Source: CAD feature listing. Evaluate the final solid. Frame: model axes, mm. A direction names the side the tool comes from. Coordinates: 2 decimals unless noted, no trailing zeros. Write each loop counter-clockwise with the first axis right and the second up, starting at its lowest first coordinate (ties: lowest second). Pieces come first, ordered by that corner, then holes. Notation, with made-up numbers: M 85.25,-15 L 117.25,-15 A19 cw 117.25,-7 Z; hole C 1,41 d4. An arc over 180 degrees is marked long. Write item = value, one per line. Start each with the question number.
1. Access query for faces 1 (the face through (-43.714, 6.409, -23.412)), 2 (the face through (-38, 6, -17.55)), 3 (the face through (-47.6, 7, -6)). Directions: +Z, -Z, +X, -X, +Y, -Y. A direction counts if a zero-diameter tool reaches every point of the face in a straight line with its end or side. Return the directions, or none.
2. Section query A-A (z = 23.75). Output: boundary loops of the cut face in (x, y).
3. Pull-direction query (X, two-part tool) for faces 4 (the face through (-43.714, 6.409, 24.088)), 5 (the face through (-44, 12, 0)), 6 (the face through (-47.6, 7, 5)); classes: pulls with the +X half, pulls with the -X half, needs draft (parallel to the pull), parting line crosses it, or undercut.
4. Pin query (flat end, axial travel): pin 1 Ø6.5 at (y, z) = (5, -6) entering from +X; pin 2 Ø4.5 at (x, z) = (-41.14, -23.75) entering from +Y; pin 3 Ø1 at (x, y) = (-43, 2.5) entering from +Z; pin 4 Ø3 at (y, z) = (10, 5.5) entering from -X. Return the tip coordinate at first contact, or that it passes through.
5. Section query D-D (x = -46.5). Output: boundary loops of the cut face in (y, z), then the cut area to 3 significant figures.
6. Line query: line 1 along Z through (x, y) = (-41, 9); line 2 along Z through (x, y) = (-42.75, 7.75); line 3 along Y through (x, z) = (-42.75, 3). Output: solid intervals per line, ascending.
7. Section query C-C (y = 4). Output: boundary loops of the cut face in (x, z), then the cut area to 3 significant figures.
8. Section query B-B (x = -39.25). Output: boundary loops of the cut face in (y, z), then the cut area to 3 significant figures.
```python
from build123d import *

# Parameters (mm, degrees)
SKETCH_1_R          = 2.6
EXTRUDE_1_DEPTH     = 13
SKETCH_2_W          = 0.6
SKETCH_2_H          = 35.1
CUT_EXTRUDE_1_DEPTH = 23
CUT_EXTRUDE_2_DEPTH = 6


with BuildPart() as part:
    # 草图1 → 凸台-拉伸1 (new body)
    with BuildSketch(Plane(origin=(0, 0, 0), x_dir=(1, 0, 0), z_dir=(0, 1, 0))):
        with BuildLine():
            Line((-33.760275315, -17.55), (-41, -17.55))
            Line((-41, -17.55), (-41, 17.55))
            Line((-41, 17.55), (-33.760275315, 17.55))
            ThreePointArc((-33.760275315, 17.55), (-36.796000438, 25.438985546), (-40.910253672, 32.823065739))
            ThreePointArc((-40.910253672, 32.823065739), (-52.45, 0), (-40.910253672, -32.823065739))
            ThreePointArc((-40.910253672, -32.823065739), (-36.796000438, -25.438985546), (-33.760275315, -17.55))
        make_face()
        with Locations(Location((-41.13620668, -23.75, 0), (0, 0, 90))):
            Circle(SKETCH_1_R, mode=Mode.SUBTRACT)
        with Locations(Location((-41.13620668, 23.75, 0), (0, 0, 90))):
            Circle(SKETCH_1_R, mode=Mode.SUBTRACT)
        with Locations(Location((-47.5, 0, 0), (0, 0, 90))):
            Circle(SKETCH_1_R, mode=Mode.SUBTRACT)
    extrude(amount=EXTRUDE_1_DEPTH)

    # 草图2 → 切除-拉伸1 (cut)
    with BuildSketch(Plane(origin=(0, 13, 0), x_dir=(1, 0, 0), z_dir=(0, 1, 0))):
        with Locations((-41.3, 0)):
            Rectangle(SKETCH_2_W, SKETCH_2_H)
    extrude(amount=-CUT_EXTRUDE_1_DEPTH, mode=Mode.SUBTRACT)

    # 草图3 → 切除-拉伸2 (cut)
    with BuildSketch(Plane(origin=(-41.6, 0, 0), x_dir=(0, 0, -1), z_dir=(1, 0, 0))):
        with BuildLine():
            Line((-5, 12), (5, 12))
            ThreePointArc((5, 12), (10, 7), (5, 2))
            Line((5, 2), (-5, 2))
            ThreePointArc((-5, 2), (-10, 7), (-5, 12))
        make_face()
    extrude(amount=-CUT_EXTRUDE_2_DEPTH, mode=Mode.SUBTRACT)


solid = part.part
```
Results are:
q1.face_1 = +Y, -Y
q1.face_2 = +X, +Y, -Y
q1.face_3 = +X
q2.outline = M -46.76,0 L -43.74,0 L -43.74,13 L -46.76,13 Z; M -38.54,0 L -36.04,0 L -36.04,13 L -38.54,13 Z
q3.face_4 = undercut
q3.face_5 = needs draft
q3.face_6 = pulls with the +X half
q4.pin_1 = -41.6
q4.pin_2 = through
q4.pin_3 = 30.74
q4.pin_4 = -52.3
q5.outline = M 0,-24.26 L 13,-24.26 L 13,-2.4 L 12,-2.4 L 12,-5 A5 cw 2,-5 L 2,-2.4 L 0,-2.4 Z; M 0,2.4 L 2,2.4 L 2,5 A5 cw 12,5 L 12,2.4 L 13,2.4 L 13,24.26 L 0,24.26 Z
q5.area = 438 mm^2
q6.line_1 = -32.71 to -26.35, -21.15 to -17.55, 17.55 to 21.15, 26.35 to 32.71
q6.line_2 = -30.39 to -25.79, -21.71 to -9.94, 9.94 to 21.71, 25.79 to 30.39
q6.line_3 = 0 to 2, 12 to 13
q7.outline = M -47.6,-9 L -47.6,-2.6 A2.6 cw -47.6,2.6 L -47.6,9 L -41.6,9 L -41.6,17.55 L -33.76,17.55 A60 ccw -40.91,32.82 A52.45 ccw -40.91,-32.82 A60 ccw -33.76,-17.55 L -41.6,-17.55 L -41.6,-9 Z; hole C -41.14,-23.75 d5.2; hole C -41.14,23.75 d5.2
q7.area = 455 mm^2
q8.outline = M 0,-30.13 L 13,-30.13 L 13,-25.54 L 0,-25.54 Z; M 0,-21.96 L 13,-21.96 L 13,-17.55 L 0,-17.55 Z; M 0,17.55 L 13,17.55 L 13,21.96 L 0,21.96 Z; M 0,25.54 L 13,25.54 L 13,30.13 L 0,30.13 Z
q8.area = 234 mm^2
